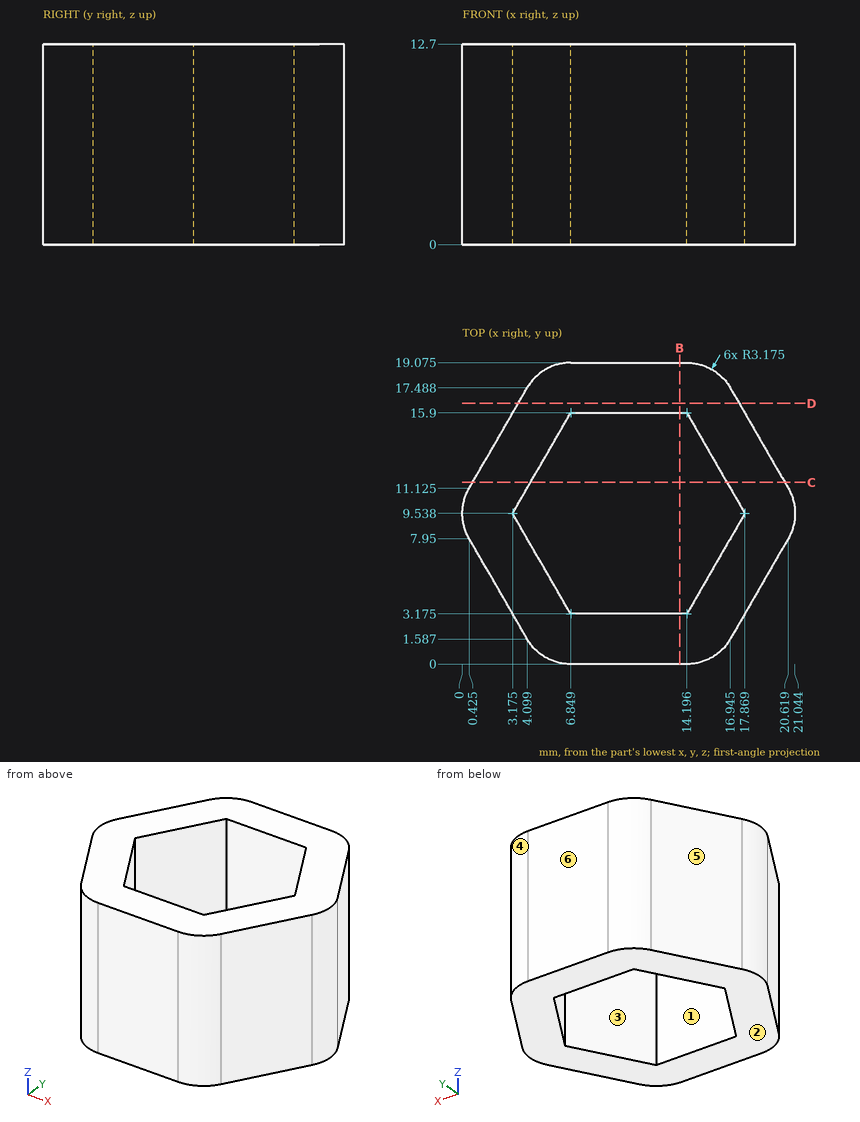
Study the drawing (mm; zero at the part's minimum x, y, z) and answer. A direction names the side the tool comes from. Give positions to 0.01 mm unless a question says otherwise; leave off trailing zeros. Write each loop counter-clockwise with the first axis right and the second up, starting at its lowest first coordinate (ties: lowest second). Pieces come first, ordered by that corner, then holes. Notation, with made-up numbers: (19, -6) - (61, -6) arc R13 ccw to (61, 19) - close; hole circle Ø3 at (-6.75, 65). An arc over 180 degrees is marked (long way). One line per question, with ' | ' between items. Start each with the question number.
1. Given P1, Ø1.5, axis at x = 3.5, z = 9.5, coming from the +Y side (1 decimal); P2, Ø4, axis at y = 12.5, z = 1.5, coming from the -X side; P3, Ø2, axis at x = 6, y = 7, coming from the +Z side, each flat-ended and moving along its own axis, determine where each tip first touches the part or whether it passes through.
2. Section D-D, the plane y = 16.5 is taken. Determine the outline of the cut face in (x, z) (1 decimal).
3. Section C-C, the plane y = 11.5 is taken. Determine the outline of the cut face in (x, z).
4. Straight lines are drawn through the part: line 1 (Y direction, x = 10.75, z = 10) (1 decimal); line 2 (Y direction, x = 17, z = 1) (1 decimal); line 3 (X direction, y = 6.75, z = 4.5) (1 decimal). For each, find the intervals that lie inside material, in ascending order.
5. Determine the mould class of the marked faces 3, 4, 5 and 6 for opening direction X: +X half, -X half, draft (parallel to the pull), parting line (faces both ways), or undercut.
6. Section B-B, the plane x = 13.75 is taken. Determine the outline of the cut face in (y, z) (1 decimal).
7. For the marked faces 1 and 2, determine the directions among +Z, -Z, +X, -X, +Y, -Y from which every point of the face is accessible in a straight line to the end or side of a thin tool.
Result:
1) P1: stops at y = 17.7 | P2: stops at x = 0.15 | P3: passes through
2) outline: (3.5, 0) - (17.5, 0) - (17.5, 12.7) - (3.5, 12.7) - close
3) outline: (0.64, 0) - (4.31, 0) - (4.31, 12.7) - (0.64, 12.7) - close; (16.74, 0) - (20.4, 0) - (20.4, 12.7) - (16.74, 12.7) - close
4) line 1: y = 0 to 3.2, 15.9 to 19.1 | line 2: y = 1.7 to 8, 11 to 17.4 | line 3: x = 1.1 to 4.8, 16.3 to 19.9
5) face 3: undercut | face 4: +X half | face 5: -X half | face 6: draft
6) outline: (0, 0) - (3.2, 0) - (3.2, 12.7) - (0, 12.7) - close; (15.9, 0) - (19.1, 0) - (19.1, 12.7) - (15.9, 12.7) - close
7) face 1: +Z, -Z | face 2: -Z, +X, -X, +Y, -Y
